The drawing under review shows one solid part. Ordinate dimensions are in mm from its lowest x, y, z. A direction names the side the tool comes from. Coordinates: 2 decimals unless noted, no trailing zeros. Write each loop counter-clockwise with the first axis right and the second up, starting at its lowest first coordinate (ties: lowest second). Pieces come first, ordered by that corner, then holes.
1) For line 1 (Z direction, x = 12, y = 21.5); line 2 (Y direction, x = 19.25, z = 78.5); line 3 (Z direction, x = 1.25, y = 6.5), list the stretches that pass through material, from the lowest coordinate up.
2) Add section A-A, the plane x = 8.5. State the section outline as (y, z) points, then the cut area to 3 significant figures.
3) Add section B-B, the plane z = 139.5. State the section outline as (x, y) points.
4) Machinability: for the marked faces 1, 2 and 3, which of the approach directions +Z, -Z, +X, -X, +Y, -Y give a long, thin tool a straight path to every point of the face, cutting with its end or side? Answer none if there is none.
5) Add section C-C, the plane y = 17.5. State the section outline as (x, z) points.
6) For P1, Ø8, axis at x = 8, z = 58.5, coming from the -Y side; P2, Ø4.5, axis at x = 10.5, y = 11.5, coming from the +Z side; P3, Ø5, axis at x = 14, z = 56.5, coming from the +Y side, all flat-tipped, find the tip position at first contact; note any pin that passes through.
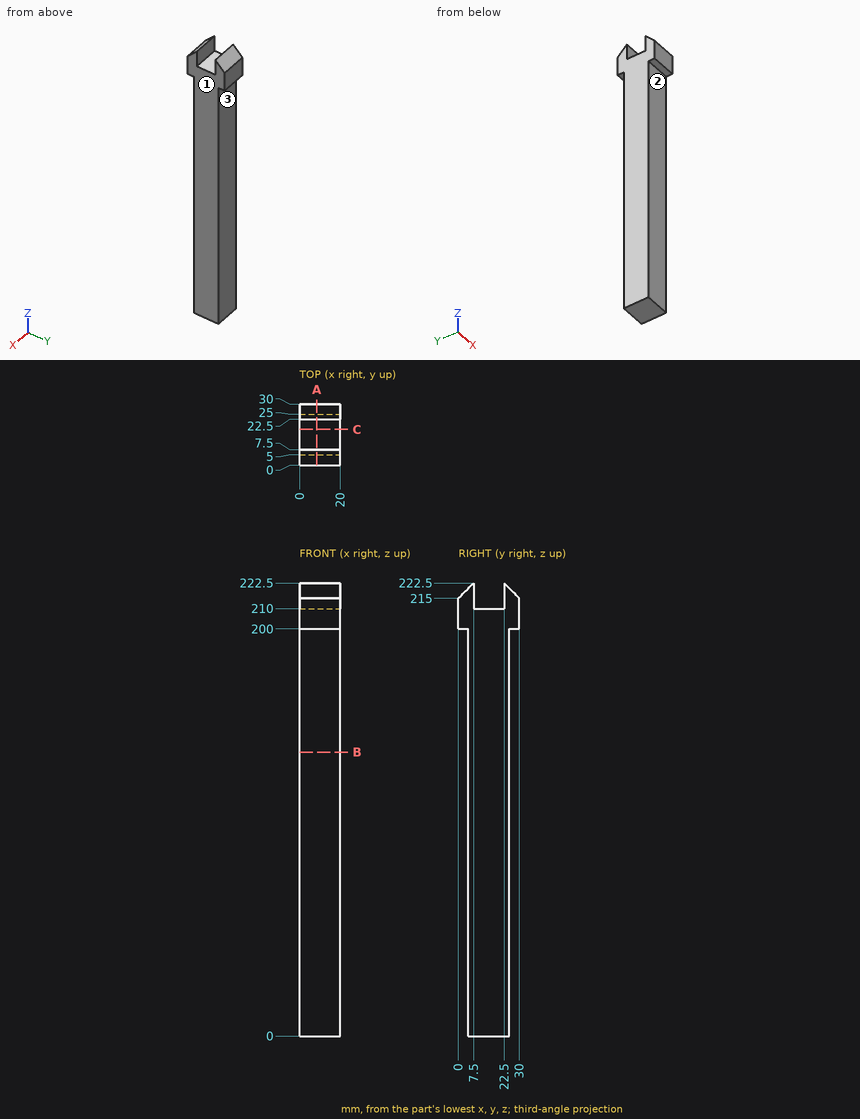
Geometry results:
1. line 1: z = 0 to 210
1. line 2: y = 5 to 25
1. line 3: z = 0 to 221.5
2. outline: (0, 200) - (5, 200) - (5, 0) - (25, 0) - (25, 200) - (30, 200) - (30, 215) - (22.5, 222.5) - (22.5, 210) - (7.5, 210) - (7.5, 222.5) - (0, 215) - close
2. area: 4,430 mm2
3. outline: (0, 5) - (20, 5) - (20, 25) - (0, 25) - close
4. face 1: +Z, -Z, +X, +Y, -Y
4. face 2: -Z, +X, -X, -Y
4. face 3: -Z, +X, -X, +Y
5. outline: (0, 0) - (20, 0) - (20, 210) - (0, 210) - close
6. P1: stops at y = 5
6. P2: stops at z = 210
6. P3: stops at y = 25
